Design review of the part shown in the three views and the two pictorial views. Dimensions are in mm from the part's minimum x, y and z. A direction names the side the tool comes from. Round coordinates to 2 decimals unless told otherwise and drop trailing zeros. Order: outer loops, then holes, each group sorted by start corner. A loop starts at its lowest first (then second) coordinate and runs counter-clockwise, first axis right, second up. Notation, with made-up numbers: (10, -35) -> (53, -35) arc R17 cw to (53, -9) -> close; hole circle Ø7 at (11, 3.25). An arc over 180 degrees is marked (long way). Put each result on its own line as item: value. Start each with the question number.
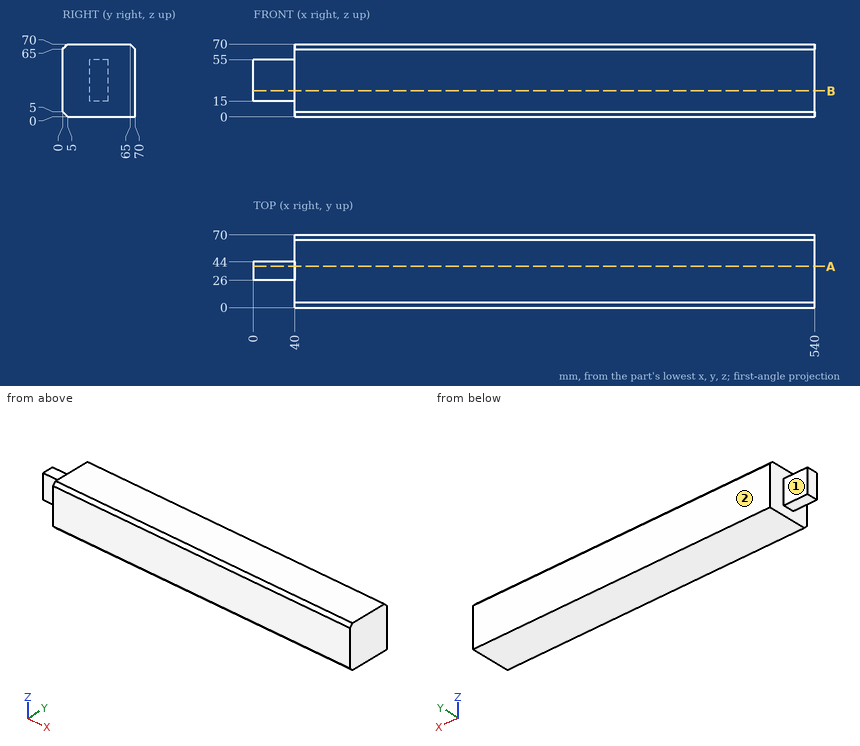
Q1. For the marked faces 1 and 2, list the 3-axis set-ups (+Z, -Z, +X, -X, +Y, -Y) from which the entire face can be reached by the end or side of a thin tool; tool diameter is ignored.
Q2. Clearance check with flat-ended pins moving along their axes: pin 1 Ø6 at (x, y) = (424.5, 46.5) entering from -Z; pin 2 Ø5 at (y, z) = (51.5, 31.5) entering from -X; pin 3 Ø12 at (x, z) = (17.5, 31.5) entering from -Y; pin 4 Ø5.5 at (x, y) = (19.5, 39) entering from +Z. State where each tip first meets the part, or that it passes through.
Q3. Take a section at B-B on z = 25. Give the boundary of the cut face in (x, y), and give its area (3 significant figures).
Q4. Take a section at A-A on y = 39.5. Give the boundary of the cut face in (x, z).
Q5. Wall thickness on probe 1 along X at (y, z) = (50, 61); probe 2 along Y at (x, z) = (80.5, 66): over which ranges is each line inside the solid? List them lowest first. Write a range as [from, to].
Calculated:
1. face 1: +Z, -Z, -X, +Y
1. face 2: +Z, -Z, +X, -X, +Y
2. pin 1: stops at z = 0
2. pin 2: stops at x = 40
2. pin 3: stops at y = 26
2. pin 4: stops at z = 55
3. outline: (0, 26) -> (40, 26) -> (40, 0) -> (540, 0) -> (540, 70) -> (40, 70) -> (40, 44) -> (0, 44) -> close
3. area: 35,700 mm²
4. outline: (0, 15) -> (40, 15) -> (40, 0) -> (540, 0) -> (540, 70) -> (40, 70) -> (40, 55) -> (0, 55) -> close
5. probe 1: x = [40, 540]
5. probe 2: y = [1, 69]
